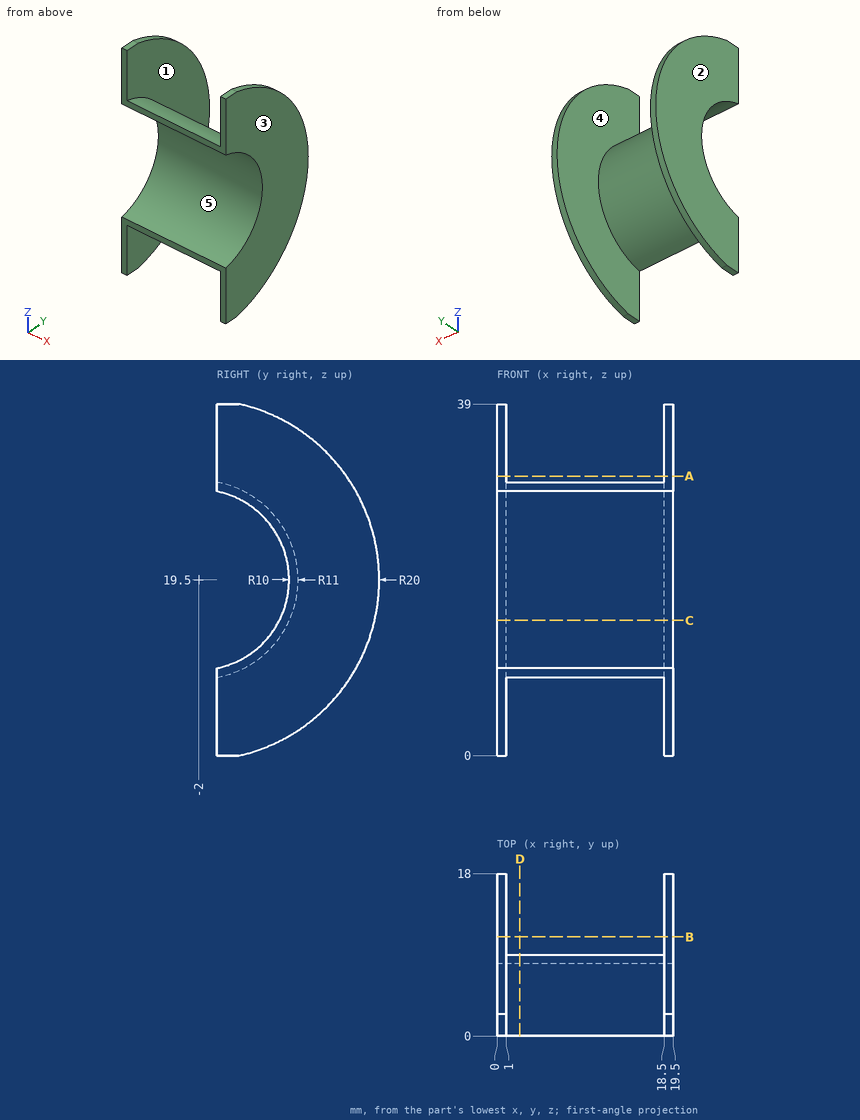
Job drawing, mm, ordinate dimensions from the low corner. One solid piece. A direction names the side the tool comes from. Coordinates: 2 decimals unless noted, no trailing zeros. Write each loop counter-clockwise with the first axis right and the second up, starting at its lowest first coordinate (ties: lowest second). Pieces come first, ordered by that corner, then holes. Notation, with made-up numbers: M 87.25,82.25 L 113.25,82.25 A3 ccw 113.25,87.25 Z; hole C 82.25,5.25 d8. An arc over 180 degrees is marked long. Answer as a JSON object with one key per item and string values. Group by question number.
1) Saw through at A-A (z = 31). Write the cut outline in (x, y), plus the area to 3 significant figures.
2) Pin check, flat tips, straight feed: pin 1 Ø1.5 at (x, y) = (13.5, 8.5) entering from -Z; pin 2 Ø1.5 at (y, z) = (4, 13) entering from -X; pin 3 Ø5 at (x, y) = (4.5, 6) entering from -Z. Stop position of each tip, or through.
3) Saw through at B-B (y = 11). Write the cut outline in (x, z), plus the area to 3 significant figures.
4) Wall check: line 1 (X direction, y = 16.75, z = 18.5); line 2 (Z direction, x = 2.75, y = 1.5); line 3 (Z direction, x = 16.5, y = 2.75). Give the ranges that are in metal, low to high. Write a range as from..to.
5) Mould opens along X. For the marked faces 1, 2 and 3 say: +X half, -X half, draft (parallel to the pull), parting line (faces both ways), or undercut.
6) Saw through at C-C (z = 15). Write the cut outline in (x, y).
7) Tool access for the marked faces 4 and 5: list every direction of +Z, -Z, +X, -X, +Y, -Y with a clear straight run to the whole face (end or side of a thin tool).
8) Saw through at D-D (x = 2.5). Write the cut outline in (y, z), plus the area to 3 significant figures.
Values follow:
{
 "1": {"outline": "M 0,0 L 1,0 L 1,14.36 L 0,14.36 Z; M 18.5,0 L 19.5,0 L 19.5,14.36 L 18.5,14.36 Z", "area": "28.7 mm2"},
 "2": {"pin 1": "stops at z = 14.41", "pin 2": "passes through", "pin 3": "stops at z = 9.97"},
 "3": {"outline": "M 0,4.3 L 1,4.3 L 1,34.7 L 0,34.7 Z; M 18.5,4.3 L 19.5,4.3 L 19.5,34.7 L 18.5,34.7 Z", "area": "60.8 mm2"},
 "4": {"line 1": "x = 0..1, 18.5..19.5", "line 2": "z = 9.07..10.13, 28.87..29.93", "line 3": "z = 9.58..10.7, 28.3..29.42"},
 "5": {"face 1": "undercut", "face 2": "-X half", "face 3": "+X half"},
 "6": {"outline": "M 0,6.93 L 19.5,6.93 L 19.5,17.49 L 18.5,17.49 L 18.5,8.04 L 1,8.04 L 1,17.49 L 0,17.49 Z"},
 "7": {"face 4": "+Y", "face 5": "+X, -X, -Y"},
 "8": {"outline": "M 0,8.68 A11 ccw 0,30.32 L 0,29.3 A10 cw 0,9.7 Z", "area": "29.0 mm2"}
}
